Could you check a few things on this model? Use its own coordinates, in mm. A direction names the side the tool comes from. Give positions to 0.01 mm unless a question says otherwise; leave off trailing zeros. Order: outer loops, then holes, each group sorted by start corner. A loop starts at its lowest first (then second) coordinate and runs counter-clockwise, first axis right, second up. Notation, with made-up numbers: M 62,7.25 L 118,7.25 A37 cw 118,43.25 Z; hole C 0.5,-38 d11. An arc over 180 degrees is marked long. Use a Markdown table: item, result. Add a question column.
Item 1: I'm going to push a flat-ended pin straight in: pin 1 Ø2.5 at (x, z) = (40.05, -10.32) entering from -Y. Where does the tip first touch, or does it pass through?
Item 2: Suppose I cut it at B-B on y = 35. Count the separate pieces of the cut face and the enclosed holes in it, plus the area to 3 significant figures.
Item 3: If we mould it in two halves opening along Y, with no side actions, what happens to faces 3 (the face through (42.79, 37.03, -27.99)), 4 (the face through (76.31, 1.01, -8.74)), 5 (the face through (44, 45, -1))? For each: released by +Y, released by -Y, zero draft, split by the parting line, or undercut.
Item 4: If I drill on L1, parallel to Z at x = 33, y = 36.5; L2, parallel to Y at x = 45, z = -1.4; L3, parallel to Y at x = 52.5, z = -8.75, over which ranges is the centre line in solid material (lowest first)? Write a range as from..to.
Item 5: Suppose I cut it at D-D on x = 67.5. Write out the boundary of the cut face in (y, z).
Item 6: For faces 1 (the face through (44, 23, -2)), 2 (the face through (83.76, 39.037, -1.014)), which set-ups out of +Z, -Z, +X, -X, +Y, -Y let a thin tool reach every point of the face, with its end or its side?
Item 7: Suppose I cut it at C-C on z = -14.5. Write out the boundary of the cut face in (x, y), plus the area to 3 significant figures.
Item 8: Suppose I cut it at A-A on x = 80. Write out the boundary of the cut face in (y, z), plus the area to 3 significant figures.
from build123d import *

# Parameters (mm, degrees)
SKETCH_1_W          = 90
SKETCH_1_H          = 29
EXTRUDE_1_DEPTH     = 2
SKETCH_4_R          = 3
SKETCH_4_R_2        = 1.5
CUT_EXTRUDE_1_DEPTH = 2
SKETCH_2_W          = 90
SKETCH_2_H          = 2
EXTRUDE_2_DEPTH     = 43
SKETCH_5_R          = 3
SKETCH_5_R_2        = 1.5
CUT_EXTRUDE_2_DEPTH = 2


with BuildPart() as part:
    # 草图1 → 凸台-拉伸1 (new body)
    with BuildSketch(Plane(origin=(0, 0, 0), x_dir=(1, 0, 0), z_dir=(0, 1, 0))):
        with Locations((45, 14.5)):
            Rectangle(SKETCH_1_W, SKETCH_1_H)
    extrude(amount=EXTRUDE_1_DEPTH)

    # 草图4 → 切除-拉伸1 (cut)
    with BuildSketch(Plane(origin=(0, 2, 0), x_dir=(1, 0, 0), z_dir=(0, 1, 0))):
        with Locations(Location((45, 14.5, 0), (0, 0, 270))):
            Circle(SKETCH_4_R)
        with Locations(Location((49.950012223, 20.223506144, 0), (0, 0, 270))):
            Circle(SKETCH_4_R_2)
        with Locations(Location((49.949507065, 10.323986856, 0), (0, 0, 270))):
            Circle(SKETCH_4_R_2)
        with Locations(Location((40.049987777, 10.324492014, 0), (0, 0, 270))):
            Circle(SKETCH_4_R_2)
        with Locations(Location((40.050492935, 20.224011302, 0), (0, 0, 270))):
            Circle(SKETCH_4_R_2)
        with Locations(Location((80, 14.5, 0), (0, 0, 270))):
            Circle(SKETCH_4_R)
        with Locations(Location((84.950012223, 19.449507065, 0), (0, 0, 270))):
            Circle(SKETCH_4_R_2)
        with Locations(Location((75.050492935, 19.450012223, 0), (0, 0, 270))):
            Circle(SKETCH_4_R_2)
        with Locations(Location((75.049987777, 9.550492935, 0), (0, 0, 270))):
            Circle(SKETCH_4_R_2)
        with Locations(Location((84.949507065, 9.549987777, 0), (0, 0, 270))):
            Circle(SKETCH_4_R_2)
        with Locations(Location((5.050492935, 9.549987777, 0), (0, 0, 90))):
            Circle(SKETCH_4_R_2)
        with Locations(Location((14.950012223, 9.550492935, 0), (0, 0, 90))):
            Circle(SKETCH_4_R_2)
        with Locations(Location((5.049987777, 19.449507065, 0), (0, 0, 90))):
            Circle(SKETCH_4_R_2)
        with Locations(Location((10, 14.5, 0), (0, 0, 90))):
            Circle(SKETCH_4_R)
        with Locations(Location((14.949507065, 19.450012223, 0), (0, 0, 90))):
            Circle(SKETCH_4_R_2)
    extrude(amount=-CUT_EXTRUDE_1_DEPTH, mode=Mode.SUBTRACT)

    # 草图2 → 凸台-拉伸2 (add)
    with BuildSketch(Plane(origin=(0, 2, 0), x_dir=(1, 0, 0), z_dir=(0, 1, 0))):
        with Locations((45, 28)):
            Rectangle(SKETCH_2_W, SKETCH_2_H)
    extrude_2 = extrude(amount=EXTRUDE_2_DEPTH)

    # 草图5 → 切除-拉伸2 (cut)
    with BuildSketch(Plane.XY.offset(-27)):
        with Locations((45, 35)):
            Circle(SKETCH_5_R)
        with Locations((49.950012223, 39.949507065)):
            Circle(SKETCH_5_R_2)
        with Locations((49.949507065, 30.049987777)):
            Circle(SKETCH_5_R_2)
        with Locations((40.049987777, 30.050492935)):
            Circle(SKETCH_5_R_2)
        with Locations((40.050492935, 39.950012223)):
            Circle(SKETCH_5_R_2)
        with Locations((80, 35)):
            Circle(SKETCH_5_R)
        with Locations((84.950012223, 39.949507065)):
            Circle(SKETCH_5_R_2)
        with Locations((75.050492935, 39.950012223)):
            Circle(SKETCH_5_R_2)
        with Locations((75.049987777, 30.050492935)):
            Circle(SKETCH_5_R_2)
        with Locations((84.949507065, 30.049987777)):
            Circle(SKETCH_5_R_2)
        with Locations(Location((5.050492935, 30.049987777, 0), (0, 0, 180))):
            Circle(SKETCH_5_R_2)
        with Locations(Location((14.950012223, 30.050492935, 0), (0, 0, 180))):
            Circle(SKETCH_5_R_2)
        with Locations(Location((5.049987777, 39.949507065, 0), (0, 0, 180))):
            Circle(SKETCH_5_R_2)
        with Locations(Location((10, 35, 0), (0, 0, 180))):
            Circle(SKETCH_5_R)
        with Locations(Location((14.949507065, 39.950012223, 0), (0, 0, 180))):
            Circle(SKETCH_5_R_2)
    cut_extrude_2 = extrude(amount=-CUT_EXTRUDE_2_DEPTH, mode=Mode.SUBTRACT)

    # 镜向1: 凸台-拉伸2, 切除-拉伸2 across plane
    add(extrude_2.mirror(Plane(origin=(0, 0, -14.5), x_dir=(1, 0, 0), z_dir=(0, 0, -1))))
    add(cut_extrude_2.mirror(Plane(origin=(0, 0, -14.5), x_dir=(1, 0, 0), z_dir=(0, 0, -1))), mode=Mode.SUBTRACT)


solid = part.part
Findings below:
| question | item | result |
|---|---|---|
| 1 | pin 1 | passes through |
| 2 | separate pieces | 8 |
| 2 | enclosed holes | 0 |
| 2 | area | 288 mm^2 |
| 3 | face 3 | undercut |
| 3 | face 4 | zero draft |
| 3 | face 5 | released by +Y |
| 4 | L1 | z = -29..-27, -2..0 |
| 4 | L2 | y = 0..32, 38..45 |
| 4 | L3 | y = 0..2 |
| 5 | outline | M 0,-29 L 45,-29 L 45,-27 L 2,-27 L 2,-2 L 45,-2 L 45,0 L 0,0 Z |
| 6 | face 1 | +X, -X, +Y |
| 6 | face 2 | +Z, -Z |
| 7 | outline | M 0,0 L 7,0 L 7,2 L 0,2 Z; M 13,0 L 42,0 L 42,2 L 13,2 Z; M 48,0 L 77,0 L 77,2 L 48,2 Z; M 83,0 L 90,0 L 90,2 L 83,2 Z |
| 7 | area | 144 mm^2 |
| 8 | outline | M 0,-29 L 32,-29 L 32,-27 L 2,-27 L 2,-17.5 L 0,-17.5 Z; M 0,-11.5 L 2,-11.5 L 2,-2 L 32,-2 L 32,0 L 0,0 Z; M 38,-29 L 45,-29 L 45,-27 L 38,-27 Z; M 38,-2 L 45,-2 L 45,0 L 38,0 Z |
| 8 | area | 194 mm^2 |
